Here's how the part is built. I have some questions about the finished solid (model axes, mm). A direction names the side the tool comes from. Give positions to 0.01 mm unless a question says otherwise; leave off trailing zeros. Loops run counter-clockwise (first coordinate to the right, second up) from the corner with the lowest first, then second, coordinate; pieces in that order, holes last. Notation, with made-up numbers: M 11.25,29.5 L 56.25,29.5 A22 cw 56.25,50.5 Z; hole C 48.25,-18.5 d1. An arc over 180 degrees is marked long. Write item = value, one per line. Start each with the question number.
```python
from build123d import *

# Parameters (mm, degrees)
SKETCH1_R           = 3.25
BOSS_EXTRUDE1_DEPTH = 3


with BuildPart() as part:
    # Sketch1 → Boss-Extrude1 (new body)
    with BuildSketch(Plane.XY):
        Polygon((4.245252181, 5.778256787), (4.245252181, 26.278256787), (18.745252181, 26.278256787), (18.745252181, 5.969156991), (18.745252181, 5.778256787), (15.995252181, 5.778256787), (15.995252181, 8.778256787), (12.995252181, 8.778256787), (12.995252181, 5.778256787), (9.995252181, 5.778256787), (9.995252181, 8.778256787), (6.995252181, 8.778256787), (6.995252181, 5.778256787), align=None)
        with Locations((11.495252181, 19.278256787)):
            Circle(SKETCH1_R, mode=Mode.SUBTRACT)
    extrude(amount=BOSS_EXTRUDE1_DEPTH)


solid = part.part
```
Q1. We'd pull the mould along X, two halves only. Please class faces 3 (the flat face through (6.995, 7, 1)), 4 (the flat face through (15.995, 7, 1)), 5 (the flat face through (13, 16, 0)), 6 (the flat face through (4.245, 16, 1)): pulls with the +X half, pulls with the -X half, needs draft (parallel to the pull), parting line crosses it, or undercut.
Q2. If we section it at C-C, the plane z = 1.3: List the corners of the cut face in (x, y) for me.
Q3. If we section it at B-B, the plane y = 20.5: List the corners of the cut face in (x, z) for me, then the cut area to 3 significant figures.
Q4. If we section it at A-A, the plane x = 11.5: List the corners of the cut face in (y, z) for me, then the cut area to 3 significant figures.
Q5. On a 3-axis mill with a long thin cutter (end or side, diameter ignored), from which of +Z, -Z, +X, -X, +Y, -Y can I reach the whole of each face in a straight line? I mean faces 1 (the flat face through (6, 5.778, 1)), 2 (the flat face through (9, 8.778, 1)). Say none if no direction works.
Q6. Will this pin go through, and if not, where does the flat tip stop? pin 1 (4 mm diameter, centred on x = 15.5, y = 8.5, fed in from +Z).
Q7. If I drill on line 1 along X through (y, z) = (8, 0.5); line 2 along X through (y, z) = (18.5, 2.75); line 3 along Y through (x, z) = (8, 1.1), over which ranges is the centre line in solid material (lowest first)?
Resolved:
q1.face_3 = undercut
q1.face_4 = undercut
q1.face_5 = needs draft
q1.face_6 = pulls with the -X half
q2.outline = M 4.25,5.78 L 7,5.78 L 7,8.78 L 10,8.78 L 10,5.78 L 13,5.78 L 13,8.78 L 16,8.78 L 16,5.78 L 18.75,5.78 L 18.75,26.28 L 4.25,26.28 Z; hole C 11.5,19.28 d6.5
q3.outline = M 4.25,0 L 8.48,0 L 8.48,3 L 4.25,3 Z; M 14.51,0 L 18.75,0 L 18.75,3 L 14.51,3 Z
q3.area = 25.4 mm²
q4.outline = M 5.78,0 L 16.03,0 L 16.03,3 L 5.78,3 Z; M 22.53,0 L 26.28,0 L 26.28,3 L 22.53,3 Z
q4.area = 42.0 mm²
q5.face_1 = +Z, -Z, +X, -X, -Y
q5.face_2 = +Z, -Z, -Y
q6.pin_1 = 3
q7.line_1 = 4.25 to 7, 10 to 13, 16 to 18.75
q7.line_2 = 4.25 to 8.34, 14.65 to 18.75
q7.line_3 = 8.78 to 26.28
